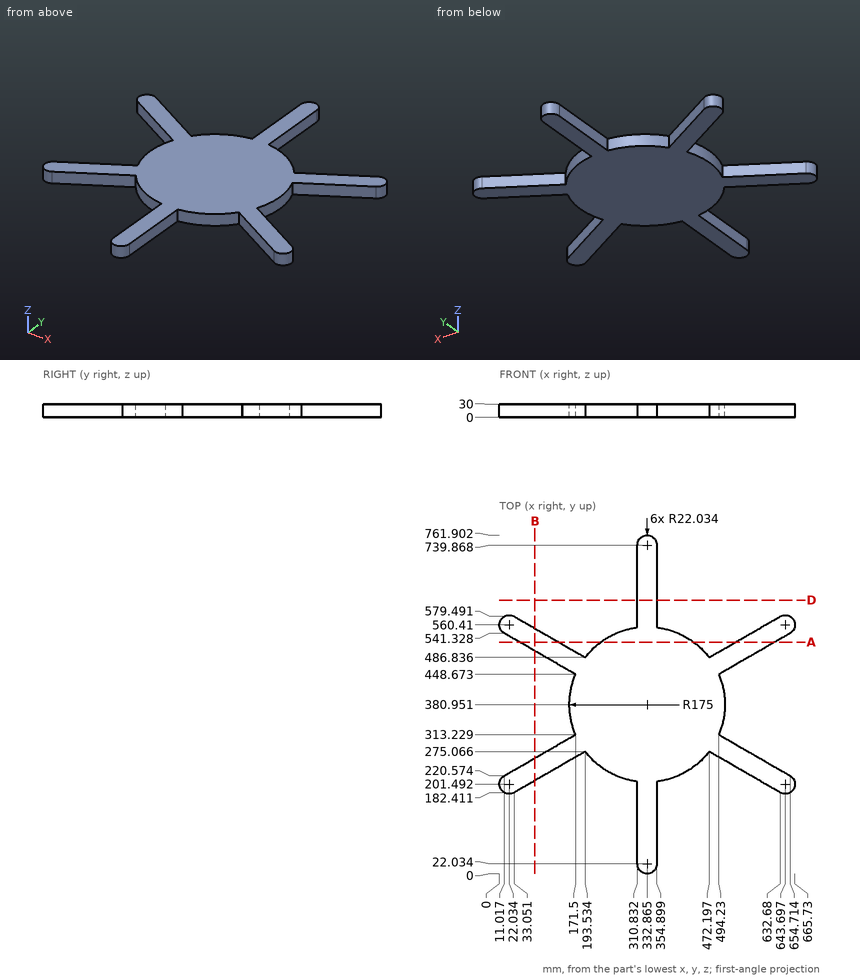
Geometry check sheet. Reference: drawing and pictorial views, mm from the part's lowest x, y, z. Coordinates: 2 decimals unless noted, no trailing zeros. Loops run counter-clockwise (first coordinate to the right, second up) from the corner with the lowest first, then second, coordinate; pieces in that order, holes last. Notation, with made-up numbers: (13, -18) - (20, -18) arc R17 cw to (20, 5) - close; hole circle Ø9 at (59.5, 5.5). An arc over 180 degrees is marked (long way). Return JSON: item names as keys, results as strings.
1. Go/stop test with flat-tipped pins: pin 1 (3 mm diameter, centred on x = 268.5, z = 4, fed in from +Y); pin 2 (9 mm diameter, centred on y = 101.5, z = 14.5, fed in from -X); pin 3 (2 mm diameter, centred on y = 370, z = 23, fed in from +X). Record where each tip stops, or that it passes through.
Established:
{"pin 1": "stops at y = 544.27", "pin 2": "stops at x = 310.83", "pin 3": "stops at x = 507.58"}
2. Section check D-D, the plane y = 616. Record the boundary of the cut face in (x, z), then the cut area to 3 significant figures.
Established:
{"outline": "(310.83, 0) - (354.9, 0) - (354.9, 30) - (310.83, 30) - close", "area": "1,320 mm2"}
3. Section check B-B, the plane x = 80. Record the boundary of the cut face in (y, z) (1 decimal), then the cut area to 3 significant figures.
Established:
{"outline": "(209.5, 0) - (260.4, 0) - (260.4, 30) - (209.5, 30) - close; (501.5, 0) - (552.4, 0) - (552.4, 30) - (501.5, 30) - close", "area": "3,050 mm2"}
4. Thickness scan on L1, parallel to Y at x = 508, z = 17.25 (1 decimal); L2, parallel to X at y = 604, z = 3.25; L3, parallel to Y at x = 622.5, z = 24.5 (1 decimal). Record the ranges inside material, lowest first.
Established:
{"L1": "y = 254.4 to 305.3, 456.6 to 507.5", "L2": "x = 310.83 to 354.9", "L3": "y = 188.3 to 239.2, 522.7 to 573.6"}
5. Section check A-A, the plane y = 521.5. Record the boundary of the cut face in (x, z) (1 decimal).
Established:
{"outline": "(45.4, 0) - (133.5, 0) - (133.5, 30) - (45.4, 30) - close; (228.6, 0) - (437.1, 0) - (437.1, 30) - (228.6, 30) - close; (532.2, 0) - (620.4, 0) - (620.4, 30) - (532.2, 30) - close"}
